from build123d import *

# Parameters (mm, degrees)
SKETCH1_R           = 1.5
BOSS_EXTRUDE1_DEPTH = 1.75
SKETCH2_W           = 10
SKETCH2_H           = 12
BOSS_EXTRUDE2_DEPTH = 6


with BuildPart() as part:
    # Sketch1 → Boss-Extrude1 (new body)
    with BuildSketch(Plane(origin=(0, 0, 0), x_dir=(1, 0, 0), z_dir=(0, 1, 0))):
        with BuildLine():
            Line((12, 11), (-12, 11))
            ThreePointArc((-12, 11), (-14.121320344, 10.121320344), (-15, 8))
            Line((-15, 8), (-15, -8))
            ThreePointArc((-15, -8), (-14.121320344, -10.121320344), (-12, -11))
            Line((-12, -11), (12, -11))
            ThreePointArc((12, -11), (14.121320344, -10.121320344), (15, -8))
            Line((15, -8), (15, 8))
            ThreePointArc((15, 8), (14.121320344, 10.121320344), (12, 11))
        make_face()
        with Locations(Location((11.5, 7.5, 0), (0, 0, 270))):
            Circle(SKETCH1_R, mode=Mode.SUBTRACT)
        with Locations(Location((11.5, -7.5, 0), (0, 0, 270))):
            Circle(SKETCH1_R, mode=Mode.SUBTRACT)
    extrude(amount=BOSS_EXTRUDE1_DEPTH)

    # Sketch2 → Boss-Extrude2 (add)
    with BuildSketch(Plane(origin=(0, 1.75, 0), x_dir=(1, 0, 0), z_dir=(0, 1, 0))):
        with Locations((-12, 0.174855127)):
            Rectangle(SKETCH2_W, SKETCH2_H)
    extrude(amount=BOSS_EXTRUDE2_DEPTH)


solid = part.part
Geometry check sheet. Reference: the model listing, model coordinates, mm. A direction names the side the tool comes from. Round coordinates to 2 decimals unless told otherwise and drop trailing zeros. Write each loop counter-clockwise with the first axis right and the second up, starting at its lowest first coordinate (ties: lowest second). Pieces come first, ordered by that corner, then holes. Notation, with made-up numbers: (1.25, -39.5) -> (6.25, -39.5) arc R10 cw to (6.25, -28.5) -> close; hole circle Ø8 at (18, -5.75). An arc over 180 degrees is marked (long way). One line per item, written item: value. Start each with the question number.
(1) Cross-section at D-D, the plane y = 3.25. Record the cut outline in (x, z).
(2) Draft check along Z on faces 1 (the cylindrical face through (14.1, 0.86, 10.14)), 2 (the cylindrical face through (11.57, 0.86, 6)), 3 (the cylindrical face through (11.57, 0.86, -9)), 4 (the flat face through (-12, 5, -6.175)). Enter one of: +Z half, -Z half, draft (parallel to the pull), parting line (faces both ways), or undercut.
(3) Cross-section at A-A, the plane x = 11.5. Record the cut outline in (y, z).
(4) Cross-section at C-C, the plane z = 7.5. Record the cut outline in (x, y).
(5) Cross-section at B-B, the plane z = -1.25. Record the cut outline in (x, y).
(6) Access from +Z, -Z, +X, -X, +Y, -Y to the whole of each face (thin tool, end or side, straight path). Record for faces 5 (the flat face through (-12, 5, 5.825)), 6 (the flat face through (-16, 1.75, 0)), 7 (the flat face through (-7, 5, 0)), 8 (the flat face through (0, 1, -11)), 9 (the flat face through (0, 0, 0)).
(7) Go/stop test with flat-tipped pins: pin 1 Ø4 at (y, z) = (4, 6) entering from +X; pin 2 Ø0.5 at (y, z) = (1, -1) entering from -X; pin 3 Ø8 at (x, z) = (3.5, -4) entering from +Y. Record where each tip stops, or that it passes through.
(8) Scan lines: line 1 (X direction, y = 0.9, z = -7.5); line 2 (Y direction, x = 0, z = 1); line 3 (X direction, y = 1.25, z = -5.25). Record each from-to range of solid material in increasing order. Write a range as [from, to].
Answer:
1. outline: (-17, -6.17) -> (-7, -6.17) -> (-7, 5.83) -> (-17, 5.83) -> close
2. face 1: +Z half
2. face 2: undercut
2. face 3: undercut
2. face 4: -Z half
3. outline: (0, -11) -> (1.75, -11) -> (1.75, -9) -> (0, -9) -> close; (0, -6) -> (1.75, -6) -> (1.75, 6) -> (0, 6) -> close; (0, 9) -> (1.75, 9) -> (1.75, 11) -> (0, 11) -> close
4. outline: (-15, 0) -> (10, 0) -> (10, 1.75) -> (-15, 1.75) -> close; (13, 0) -> (15, 0) -> (15, 1.75) -> (13, 1.75) -> close
5. outline: (-17, 1.75) -> (-15, 1.75) -> (-15, 0) -> (15, 0) -> (15, 1.75) -> (-7, 1.75) -> (-7, 7.75) -> (-17, 7.75) -> close
6. face 5: +Z, +X, -X, +Y
6. face 6: +Z, -Z, -X, -Y
6. face 7: +Z, -Z, +X, +Y
6. face 8: -Z, +X, -X, +Y, -Y
6. face 9: +Z, -Z, +X, -X, -Y
7. pin 1: x = -7
7. pin 2: x = -15
7. pin 3: y = 1.75
8. line 1: [-15, 10], [13, 15]
8. line 2: [0, 1.75]
8. line 3: [-15, 15]
